```python
from build123d import *

# Parameters (mm, degrees)
BOSS_EXTRUDE1_DEPTH = 3.175
CUT_EXTRUDE1_DEPTH  = 3.175


with BuildPart() as part:
    # Sketch1 → Boss-Extrude1 (new body)
    with BuildSketch(Plane(origin=(0, 0, 0), x_dir=(0, 0, -1), z_dir=(1, 0, 0))):
        with BuildLine():
            Line((0, 199.9996), (87.2998, 199.9996))
            ThreePointArc((87.2998, 199.9996), (99.9998, 187.2996), (112.6998, 199.9996))
            Line((112.6998, 199.9996), (199.9996, 199.9996))
            Line((199.9996, 199.9996), (199.9996, 0))
            Line((199.9996, 0), (0, 0))
            Line((0, 0), (0, 199.9996))
        make_face()
    extrude(amount=BOSS_EXTRUDE1_DEPTH)

    # Sketch2 → Cut-Extrude1 (cut)
    with BuildSketch(Plane(origin=(3.175, 0, 0), x_dir=(0, 0, -1), z_dir=(1, 0, 0))):
        with BuildLine():
            Line((199.9996, 199.9996), (112.6998, 199.9996))
            ThreePointArc((112.6998, 199.9996), (99.9998, 187.2996), (87.2998, 199.9996))
            Line((87.2998, 199.9996), (0, 199.9996))
            Line((0, 199.9996), (0, 0))
            Line((0, 0), (199.9996, 0))
            Line((199.9996, 0), (199.9996, 199.9996))
        make_face()
        with BuildLine():
            Line((199.898, 199.898), (112.800996819, 199.898))
            ThreePointArc((112.800996819, 199.898), (99.9998, 187.198), (87.198603181, 199.898))
            Line((87.198603181, 199.898), (0.1016, 199.898))
            Line((0.1016, 199.898), (0.1016, 0.1016))
            Line((0.1016, 0.1016), (199.898, 0.1016))
            Line((199.898, 0.1016), (199.898, 199.898))
        make_face(mode=Mode.SUBTRACT)
    extrude(amount=-CUT_EXTRUDE1_DEPTH, mode=Mode.SUBTRACT)


solid = part.part
```
Design review of the part built by this model. Coordinates are the model's own, in mm. Give positions to 0.01 mm unless a question says otherwise; leave off trailing zeros. Loops run counter-clockwise (first coordinate to the right, second up) from the corner with the lowest first, then second, coordinate; pieces in that order, holes last. Notation, with made-up numbers: (-27.5, 54) -> (-7.5, 54) arc R20 cw to (-7.5, 74) -> close; hole circle Ø3 at (-2.75, 13). An arc over 180 degrees is marked (long way). One line per item, written item: value.
Q1. We need section A-A on z = -97. Give the boundary of the cut face in (x, y) (3 decimals).
Numbers:
outline: (0, 0.102) -> (3.175, 0.102) -> (3.175, 187.554) -> (0, 187.554) -> close
Q2. Draft analysis for pull direction Z (two halves, no side actions). For faces 1 (the flat face through (0, 101, -101)), 2 (the cylindrical face through (1.6, 187.2, -100.3)), state which applies: pulls with the +Z half, pulls with the -Z half, needs draft (parallel to the pull), parting line crosses it, or undercut.
Numbers:
face 1: needs draft
face 2: undercut
Q3. For L1, parallel to Y at x = 2.1, z = -98; L2, parallel to Y at x = 1.65, z = -90.5, list the stretches that pass through material, from the lowest coordinate up.
Numbers:
L1: y = 0.1 to 187.36
L2: y = 0.1 to 191.42
